```python
from build123d import *

# Parameters (mm, degrees)
F0_R     = 2.5625
F1_DEPTH = 4.25
F0_R_2   = 3.75
F2_DEPTH = 1.25
F0_R_3   = 5.25
F3_DEPTH = 1
F4_R     = 0.625


with BuildPart() as f1:
    # F0 (on Top) → F1 (new body)
    with BuildSketch(Plane.XY):
        Circle(F0_R)
    extrude(amount=F1_DEPTH)

    # F0 (on Top) → F2 (join)
    with BuildSketch(Plane.XY):
        Circle(F0_R_2)
        Circle(F0_R, mode=Mode.SUBTRACT)
    extrude(amount=F2_DEPTH)

    # F0 (on Top) → F3 (join)
    with BuildSketch(Plane.XY):
        Circle(F0_R_3)
        Circle(F0_R_2, mode=Mode.SUBTRACT)
    extrude(amount=F3_DEPTH)

    # F4
    f4_edges = [f1.edges().sort_by_distance(p)[0] for p in [
        (-5.25, 0, 0),
        (-2.5625, 0, 4.25),
    ]]
    fillet(f4_edges, radius=F4_R)


solid = f1.part
```
Model file for the job. Use its own axes, mm. A direction names the side the tool comes from. Coordinates: 2 decimals unless noted, no trailing zeros. Order: outer loops, then holes, each group sorted by start corner. A loop starts at its lowest first (then second) coordinate and runs counter-clockwise, first axis right, second up. Notation, with made-up numbers: M -15,28.5 L -9,28.5 A31 cw -9,54.5 Z; hole C -19,-1 d4. An arc over 180 degrees is marked long. Answer as CSV lines item,"result".
(1) Flat gauge pins, fed straight in: pin 1 (1 mm diameter, centred on x = -2, z = 3, fed in from +Y); pin 2 (1.5 mm diameter, centred on x = 3, z = 3.5, fed in from +Y); pin 3 (2 mm diameter, centred on x = -2, z = 1.5, fed in from +Y). Where does each tip first touch, or does it go through?
Geometry says:
pin 1,"stops at y = 2.08"
pin 2,"stops at y = 1.23"
pin 3,"stops at y = 5.13"
(2) Band-saw the part on C-C, the plane z = 2.65. List the corners of the cut face in (x, y) (1 decimal).
Geometry says:
outline,"C 0,0 d5.1"
(3) 3-axis set-ups, long thin cutter, end or side, ignore diameter. For faces 1 (the flat face through (0, 0, 4.25)), 2 (the flat face through (-1, 4, 1)): which of +Z, -Z, +X, -X, +Y, -Y reach the whole face in a straight line?
Geometry says:
face 1,"+Z, +X, -X, +Y, -Y"
face 2,"+Z"
(4) Wall check: line 1 along Z through (x, y) = (0.75, 4); line 2 along Z through (x, y) = (-2.75, 0.75); line 3 along Y through (x, z) = (-0.5, 1.1). Give the ranges that are in metal, low to high.
Geometry says:
line 1,"z = 0 to 1"
line 2,"z = 0 to 1.25"
line 3,"y = -3.72 to 3.72"
